Job drawing, mm, ordinate dimensions from the low corner. One solid piece. Round coordinates to 2 decimals unless told otherwise and drop trailing zeros. Write each loop counter-clockwise with the first axis right and the second up, starting at its lowest first coordinate (ties: lowest second). Pieces come first, ordered by that corner, then holes. Notation, with made-up numbers: (-32.5, 3) - (21.5, 3) arc R22 ccw to (21.5, 14) - close; hole circle Ø9 at (-8.75, -31.5). An arc over 180 degrees is marked (long way). Write each question's results on one line, items separated by ' | '.
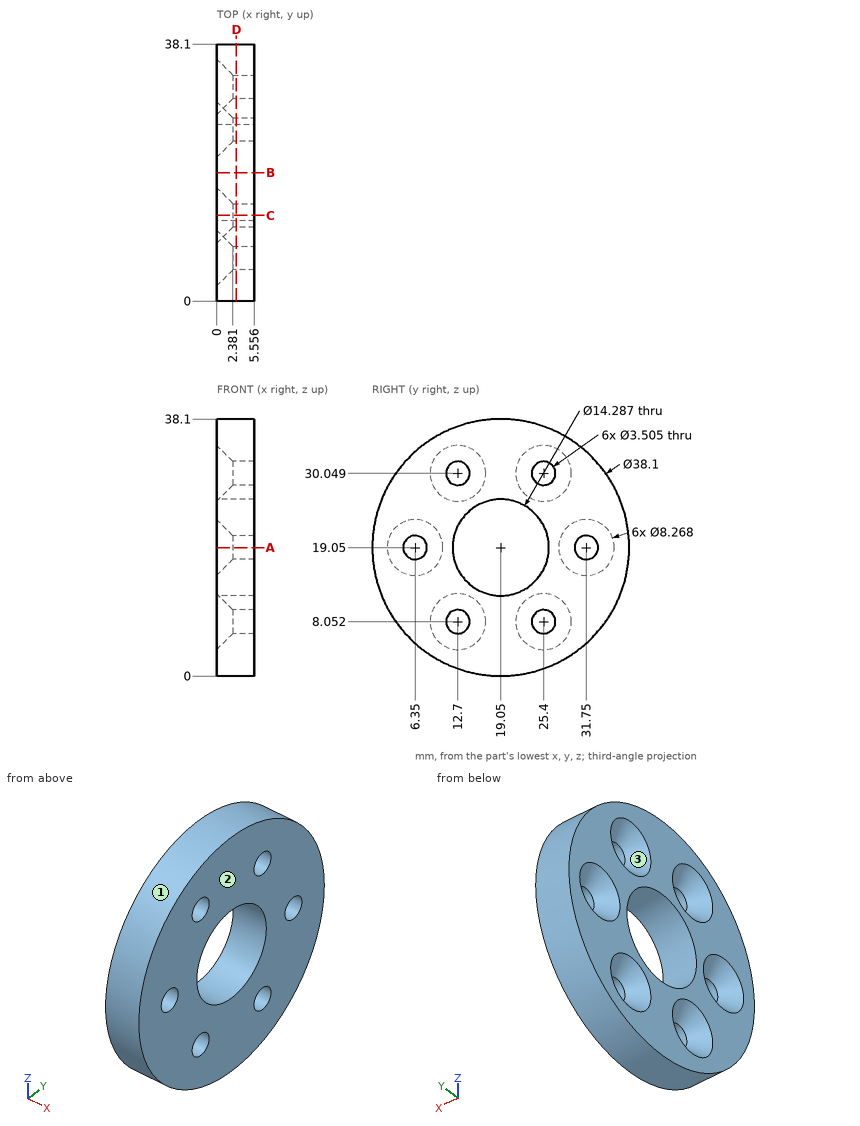
(1) Drill centre lines: probe 1 along Y at (x, z) = (0.9, 18) (1 decimal); probe 2 along Y at (x, z) = (1.55, 10) (1 decimal); probe 3 along Y at (x, z) = (5.3, 20) (1 decimal). Where is each one in solid material? Low to high. Write a range as [from, to].
Worked answers:
probe 1: y = [0, 3.3], [9.4, 12], [26.1, 28.7], [34.8, 38.1] | probe 2: y = [2.3, 11], [14.4, 23.7], [27.1, 35.8] | probe 3: y = [0, 4.9], [7.8, 12], [26.1, 30.3], [33.2, 38.1]
(2) Flat gauge pins, fed straight in: pin 1 Ø2 at (x, y) = (4, 5.5) entering from -Z; pin 2 Ø3 at (x, z) = (3, 26) entering from +Y. Where does each tip first touch, or does it go through?
Worked answers:
pin 1: stops at z = 4.72 | pin 2: stops at y = 37.3
(3) Slice it at C-C, the plane y = 12.7. Write the cut outline in (x, z) (1 decimal).
Worked answers:
outline: (0, 1.1) - (5.6, 1.1) - (5.6, 6.3) - (2.4, 6.3) - (0, 3.9) - close; (0, 12.2) - (2.4, 9.8) - (5.6, 9.8) - (5.6, 15.8) - (0, 15.8) - close; (0, 22.3) - (5.6, 22.3) - (5.6, 28.3) - (2.4, 28.3) - (0, 25.9) - close; (0, 34.2) - (2.4, 31.8) - (5.6, 31.8) - (5.6, 37) - (0, 37) - close
(4) Slice it at B-B, the plane y = 19.05. Write the cut outline in (x, z).
Worked answers:
outline: (0, 0) - (5.56, 0) - (5.56, 11.91) - (0, 11.91) - close; (0, 26.19) - (5.56, 26.19) - (5.56, 38.1) - (0, 38.1) - close
(5) Two-plate mould, pull along Z, no slides. Class the marked faces 1, 2 and 3: released by +Z, released by -Z, zero draft, split by the parting line, or undercut.
Worked answers:
face 1: split by the parting line | face 2: zero draft | face 3: undercut
(6) Slice it at A-A, the plane z = 19.05. Write the cut outline in (x, y).
Worked answers:
outline: (0, 0) - (5.56, 0) - (5.56, 4.6) - (2.38, 4.6) - (0, 2.22) - close; (0, 10.48) - (2.38, 8.1) - (5.56, 8.1) - (5.56, 11.91) - (0, 11.91) - close; (0, 26.19) - (5.56, 26.19) - (5.56, 30) - (2.38, 30) - (0, 27.62) - close; (0, 35.88) - (2.38, 33.5) - (5.56, 33.5) - (5.56, 38.1) - (0, 38.1) - close
(7) Slice it at D-D, the plane x = 2.9. State how many separate pieces and enclosed holes the cut face has, and give its area (3 significant figures).
Worked answers:
separate pieces: 1 | enclosed holes: 7 | area: 922 mm2
